```python
from build123d import *

# Parameters (mm, degrees)
F0_R      = 13
F0_R_2    = 38
F1_DEPTH  = 28
F3_R      = 30
F5_D      = 26
F6_D      = 26
F7_D      = 34
F7_DEPTH  = 28.001
F8_R      = 17
F9_DEPTH  = 25
F10_DEPTH = 35


# Not quite as in the source:
# - ends of sketch curves that miss each other by under 0.0002 mm in the source are joined


with BuildPart() as f1:
    # F0 (on Front) → F1 (new body)
    with BuildSketch(Plane.XZ):
        with BuildLine():
            Line((67.5423051658, 29.6541306361), (0, 40))
            Line((0, 40), (-67.5423051658, 29.6541306361))
            ThreePointArc((-67.5423051658, 29.6541306361), (-93, 0), (-67.5423051658, -29.6541306361))
            Line((-67.5423051658, -29.6541306361), (0, -40))
            Line((0, -40), (67.5423036859, -29.6541209752))
            ThreePointArc((67.5423036859, -29.6541209752), (67.5542752903, -29.6522946259), (67.5662446728, -29.6504537839))
            ThreePointArc((67.5662446728, -29.6504537839), (92.9999975558, 0.0121101119), (67.5423051658, 29.6541306361))
        make_face()
        with Locations((-63, 0)):
            Circle(F0_R, mode=Mode.SUBTRACT)
        Circle(F0_R_2, mode=Mode.SUBTRACT)
        with Locations((63, 0)):
            Circle(F0_R, mode=Mode.SUBTRACT)
        with Locations((-63, 0)):
            Circle(F0_R)
        Circle(F0_R_2)
        with Locations((63, 0)):
            Circle(F0_R)
    extrude(amount=-F1_DEPTH)

    # F3 (on offset) → F4 section 0
    with BuildSketch(Plane.XZ.offset(10)):
        Circle(F3_R)
    # F0 (on Front) → F4 section 1
    with BuildSketch(Plane.XZ):
        Circle(F0_R_2)
    loft()

    # F5 (through all)
    with Locations(Plane.XZ):
        with Locations((-63, 0)):
            Hole(F5_D / 2)

    # F6 (through all)
    with Locations(Plane.XZ):
        with Locations((63, 0)):
            Hole(F6_D / 2)

    # F7 (through all, one way)
    with BuildSketch(Plane.XZ):
        with Locations((0, 0)):
            Circle(F7_D / 2)
    extrude(amount=-F7_DEPTH, mode=Mode.SUBTRACT)

    # F8 (on face) → F9 (cut)
    with BuildSketch(Plane.XZ.offset(10)):
        Circle(F8_R)
    extrude(amount=-F9_DEPTH, mode=Mode.SUBTRACT)

    # F10 (add): a face of the model
    f10_faces = [f1.faces().sort_by_distance(p)[0] for p in [
        (90.975250823, 28, 0.0112927815),
    ]]
    extrude(f10_faces, amount=F10_DEPTH)


solid = f1.part
```
Source: CAD feature listing. Evaluate the final solid. Frame: model axes, mm. Coordinates: 2 decimals unless noted, no trailing zeros. Loops run counter-clockwise (first coordinate to the right, second up) from the corner with the lowest first, then second, coordinate; pieces in that order, holes last. Notation, with made-up numbers: M -0.5,43 L 9.5,43 A31 ccw 9.5,71 Z; hole C 76.25,32.25 d6. An arc over 180 degrees is marked long. Put each result on its own line as item: value. Start each with the question number.
1) Cut plane B-B on x = -63. Return the cut outline in (y, z).
2) Cut plane A-A on y = 13.5. Give the number of separate pieces and of enclosed holes in the cut face, then the cut area to 3 significant figures.
3) Contact query for flat-ended pins moving along their axis: pin 1 Ø12 at (y, z) = (7.5, -22) entering from -X; pin 2 Ø4 at (x, y) = (-6, 18.5) entering from -Z; pin 3 Ø1.5 at (x, y) = (-60.5, 0.5) entering from +Z. Output: stop coordinate, or through.
4) Ray query, L1, parallel to X at y = 33.5, z = 0.5; L2, parallel to X at y = 28.5, z = -2.5; L3, parallel to Z at x = 0, y = 7. Return the intervals inside material, ascending. Write a range as from..to.
5) Cut plane D-D on x = 64.5. Return the cut outline in (y, z).
The answers:
1. outline: M 0,-30.35 L 63,-30.35 L 63,-13 L 0,-13 Z; M 0,13 L 63,13 L 63,30.35 L 0,30.35 Z
2. separate pieces: 1
2. enclosed holes: 3
2. area: 9,720 mm²
3. pin 1: stops at x = -88.38
3. pin 2: stops at z = -39.39
3. pin 3: stops at z = 30.85
4. L1: x = -93..-75.99, -50.01..-16.99, 16.99..50.01, 75.99..93
4. L2: x = -92.9..-75.76, -50.24..-16.82, 16.82..50.24, 75.76..92.9
4. L3: z = -40..-17, 17..40
5. outline: M 0,-30.12 L 63,-30.12 L 63,-12.91 L 0,-12.91 Z; M 0,12.91 L 63,12.91 L 63,30.12 L 0,30.12 Z
